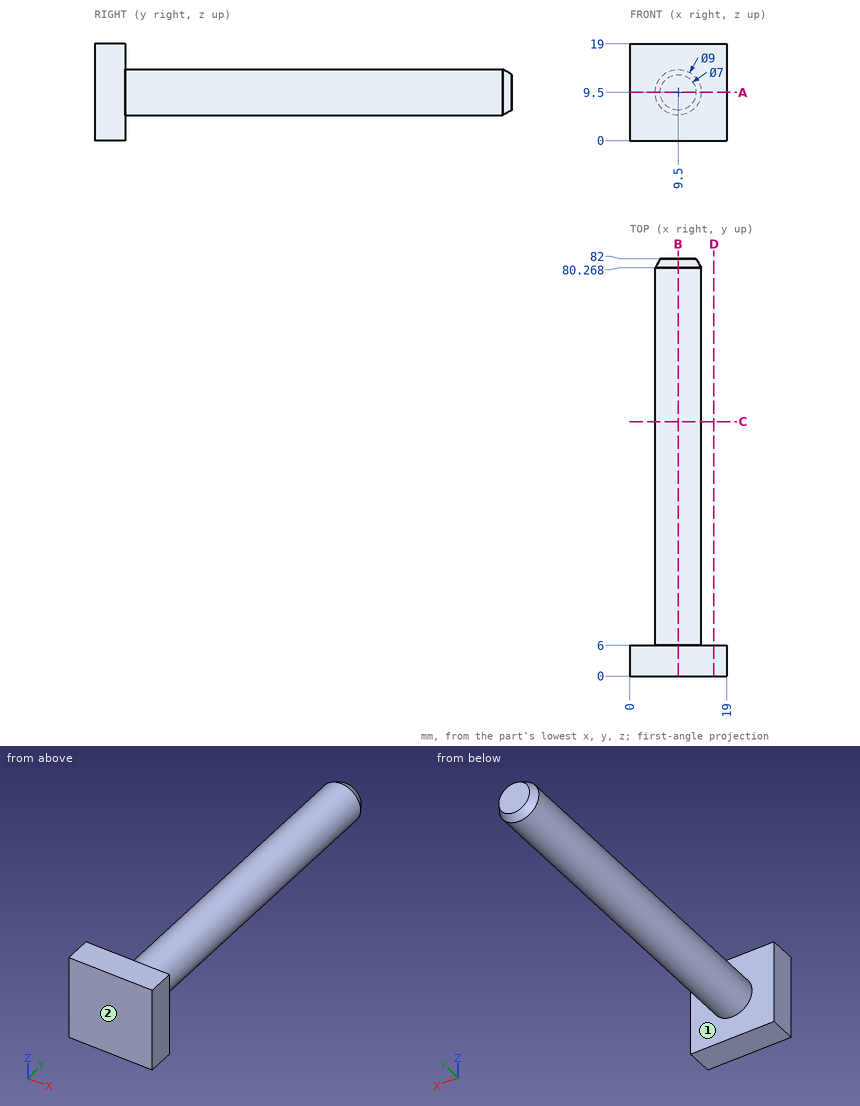
Study the drawing (mm; zero at the part's minimum x, y, z) and answer. A direction names the side the tool comes from. Give positions to 0.01 mm unless a question says otherwise; leave off trailing zeros. Order: outer loops, then holes, each group sorted by start corner. A loop starts at its lowest first (then second) coordinate and runs counter-clockwise, first axis right, second up.
1) Find section C-C on y = 50. Write down the section's boundary in (x, z), then the cut area to 3 significant figures.
Reported:
outline: circle Ø9 at (9.5, 9.5)
area: 63.6 mm2
2) Find section A-A on z = 9.5. Write down the section's boundary in (x, y).
Reported:
outline: (0, 0) - (19, 0) - (19, 6) - (14, 6) - (14, 80.27) - (13, 82) - (6, 82) - (5, 80.27) - (5, 6) - (0, 6) - close
3) Given P1, Ø10, axis at x = 14.5, y = 46, coming from the +Z side; P2, Ø5, axis at y = 48, z = 12.5, coming from the +X side; P3, Ø6, axis at y = 16, z = 4, coming from the -X side, each flat-ended and moving along its own axis, determine where each tip first touches the part or whether it passes through.
Reported:
P1: stops at z = 14
P2: stops at x = 13.97
P3: stops at x = 5.76
4) Find section D-D on x = 16.5. Write down the section's boundary in (y, z), then the cut area to 3 significant figures.
Reported:
outline: (0, 0) - (6, 0) - (6, 19) - (0, 19) - close
area: 114 mm2
5) For the marked faces 1 and 2, determine the directions among +Z, -Z, +X, -X, +Y, -Y from which every point of the face is accessible in a straight line to the end or side of a thin tool.
Reported:
face 1: +Y
face 2: +Z, -Z, +X, -X, -Y
6) Find section B-B on x = 9.5. Write down the section's boundary in (y, z), then the cut area to 3 significant figures.
Reported:
outline: (0, 0) - (6, 0) - (6, 5) - (80.27, 5) - (82, 6) - (82, 13) - (80.27, 14) - (6, 14) - (6, 19) - (0, 19) - close
area: 796 mm2
7) Consider line 1 along Y through (x, z) = (4, 16); line 2 along X through (y, z) = (75, 9.5); line 3 along X through (y, z) = (22, 8.5). Determine where each line is inside the solid, lowest interval first.
Reported:
line 1: y = 0 to 6
line 2: x = 5 to 14
line 3: x = 5.11 to 13.89
